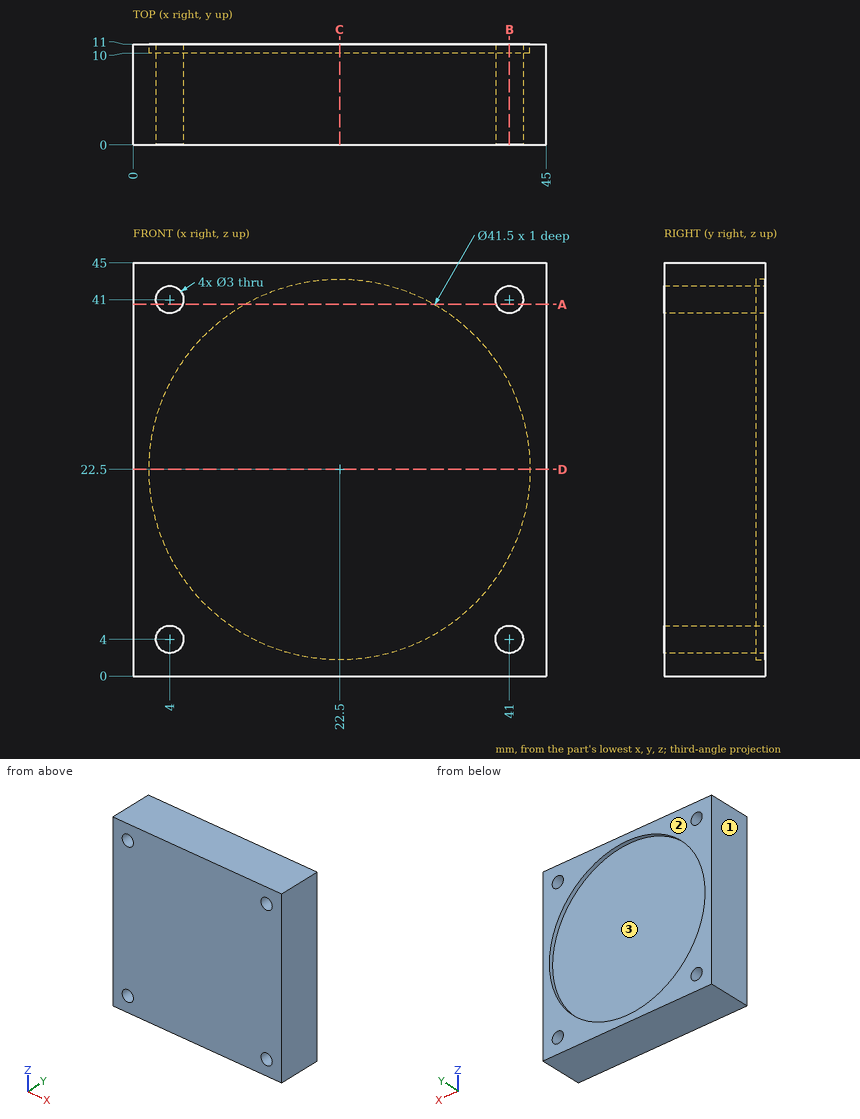
The figure shows three views and two pictorial views of one solid part (mm, origin at its lowest corner). Answer the questions. Give positions to 0.01 mm unless a question says otherwise; leave off trailing zeros. Write each loop counter-clockwise with the first axis right and the second up, starting at its lowest first coordinate (ties: lowest second). Pieces come first, ordered by that corner, then holes.
Q1. The part is cut by section B-B on x = 41. Give the vertices of the cut face in (y, z), and give its area (3 significant figures).
Answer:
outline: (0, 0) - (11, 0) - (11, 2.5) - (0, 2.5) - close; (0, 5.5) - (11, 5.5) - (11, 13.1) - (10, 13.1) - (10, 31.9) - (11, 31.9) - (11, 39.5) - (0, 39.5) - close; (0, 42.5) - (11, 42.5) - (11, 45) - (0, 45) - close
area: 410 mm2
Q2. The part is cut by section C-C on x = 22.5. Give the vertices of the cut face in (y, z), and give its area (4 significant figures).
Answer:
outline: (0, 0) - (11, 0) - (11, 1.75) - (10, 1.75) - (10, 43.25) - (11, 43.25) - (11, 45) - (0, 45) - close
area: 453.5 mm2
Q3. Given pin 1 (2.5 mm diameter, centred on x = 41, z = 41, fed in from +Y); pin 2 (1.5 mm diameter, centred on x = 18.5, z = 7, fed in from +Y), each flat-ended and moving along its own axis, determine where each tip first touches the part or whether it passes through.
Answer:
pin 1: passes through
pin 2: stops at y = 10
Q4. For a pull along X with two mould halves and no side action, classify the marked faces 1, 2 and 3 as released by +X, released by -X, zero draft, split by the parting line, or undercut.
Answer:
face 1: released by -X
face 2: zero draft
face 3: undercut
Q5. Straight lines are drawn through the part: L1, parallel to X at y = 8, z = 41; L2, parallel to X at y = 10.3, z = 22.5; L3, parallel to X at y = 10.25, z = 28. For each, find the intervals that lie inside material, in ascending order.
Answer:
L1: x = 0 to 2.5, 5.5 to 39.5, 42.5 to 45
L2: x = 0 to 1.75, 43.25 to 45
L3: x = 0 to 2.49, 42.51 to 45
Q6. The part is cut by section A-A on z = 40.5. Give the vertices of the cut face in (x, y).
Answer:
outline: (0, 0) - (2.59, 0) - (2.59, 11) - (0, 11) - close; (5.41, 0) - (39.59, 0) - (39.59, 11) - (32.82, 11) - (32.82, 10) - (12.18, 10) - (12.18, 11) - (5.41, 11) - close; (42.41, 0) - (45, 0) - (45, 11) - (42.41, 11) - close
Q7. The part is cut by section D-D on z = 22.5. Give the vertices of the cut face in (x, y).
Answer:
outline: (0, 0) - (45, 0) - (45, 11) - (43.25, 11) - (43.25, 10) - (1.75, 10) - (1.75, 11) - (0, 11) - close
